Autodesk Inventor part; units mm, degrees
ref_plane "YZ Plane" through (0, 0, 0) normal (1, 0, 0) x (0, 1, 0)
ref_plane "XZ Plane" through (0, 0, 0) normal (0, 1, 0) x (-1, 0, 0)
ref_plane "XY Plane" through (0, 0, 0) normal (0, 0, 1) x (1, 0, 0)
ref_plane "Work Plane6" through (39.7008, -57.1298, -11.5364) normal (0, 0, 1) x (1, 0, 0)
sketch "Sketch1" plane through (39.7008, -57.1298, -11.5364) normal (0, 0, 1) x (1, 0, 0)
  line L0 (-30.146, 63.9369) -> (29.7552, 63.9369)
  line L1 (29.7552, 63.9369) -> (29.7552, 15.006)
  line L2 (29.7552, 15.006) -> (-30.146, 15.006)
  line L3 (-30.146, 15.006) -> (-30.146, 63.9369)
  point P0 (-39.7008, 57.1298)
extrude "Extrusion1" add sketch "Sketch1" against normal blind 3.81
ref_plane "Work Plane5" through (9.5547, -42.1238, -11.5364) normal (0, -1, 0) x (1, 0, 0)
sketch "Sketch4" plane through (9.5547, -42.1238, -11.5364) normal (0, -1, 0) x (1, 0, 0)
  line L0 (59.9013, -3.81) -> (0, -3.81)
  line L1 (51.9539, -3.81) -> (48.6512, -3.81)
  line L2 (48.6512, -3.81) -> (48.6512, -2.9224)
  line L3 (48.6512, -2.9224) -> (51.9539, -2.9224)
  line L4 (51.9539, -2.9224) -> (51.9539, -3.81)
  line L5 (14.0976, -3.7678) -> (10.0617, -3.7678)
  line L6 (10.0617, -3.7678) -> (10.0617, -2.9224)
  line L7 (10.0617, -2.9224) -> (14.0976, -2.9224)
  line L8 (14.0976, -2.9224) -> (14.0976, -3.7678)
  point P0 (-9.5547, 11.5364)
  point P1 (48.6512, -3.81)
extrude "Extrusion2" add sketch "Sketch4" along normal blind 2.54
sketch "Sketch5" plane through (39.7008, -57.1298, -11.5364) normal (0, 0, 1) x (1, 0, 0)
  line L0 (-17.172, 70.4399) -> (-9.7142, 70.4399)
  line L1 (-9.7142, 70.4399) -> (-9.7142, 57.1298)
  line L2 (-9.7142, 57.1298) -> (-17.172, 57.1298)
  line L3 (-17.172, 57.1298) -> (-17.172, 70.4399)
  point P0 (-39.7008, 57.1298)
extrude "Extrusion3" add sketch "Sketch5" along normal blind 2.54
sketch "Sketch6" plane through (39.7008, -57.1298, -8.9964) normal (0, 0, 1) x (1, 0, 0)
  point P0 (-39.7008, 57.1298)
  point P1 (-13.4232, 67.2539)
hole "Hole1" at (26.2775, 10.1241, -8.9964) direction (0, 0, -1) diameter 2.286 end through all
properties part number "batteryFlap"
Read the model definition and answer for the solid it produces. Units are mm, in the model's axes. A direction names the side the tool comes from. Round coordinates to 2 decimals unless told otherwise and drop trailing zeros. Loops run counter-clockwise (first coordinate to the right, second up) from the corner with the lowest first, then second, coordinate; pieces in that order, holes last.
Q1. Which of the six approach directions +Z, -Z, +X, -X, +Y, -Y give full straight-line access (tool end or side, diameter ignored) to faces 1 (the face through (22.529, 7, -10)), 2 (the face through (22, -43, -14.459)), 3 (the face through (25, 9, -11.536)), 4 (the face through (29.987, 7, -10))?
Q2. Each of these flat-tipped pins is pushed along its axis until it touches: pin 1 (2 mm diameter, centred on x = 60.5, y = -44, fed in from +Z); pin 2 (0.9 mm diameter, centred on y = -44, z = -15, fed in from -X); pin 3 (1.5 mm diameter, centred on x = 30.5, z = -12, fed in from -Y); pin 4 (5 mm diameter, centred on x = 49, y = 7, fed in from -Z). Where does it stop, or does it pass through?
Q3. Section A-A on y = 1 is taken. Write down the section's boundary in (x, z).
Q4. Section B-B on z = -10.25 is taken. Write down the section's boundary in (x, y), and give its area (3 significant figures).
Q5. Determine the mould class of faces 5 (the face through (40, -42.124, -13)), 6 (the face through (25.144, 10.273, -10.284)), 7 (the face through (39, -17, -11.536)), 8 (the face through (9.555, -18, -13)) for opening direction X: released by +X, released by -X, zero draft, split by the parting line, or undercut.
Q6. Section C-C on x = 15.5 is taken. Write down the section's boundary in (y, z), and give its area (3 significant figures).
Q7. Consider probe 1 along Y at (x, z) = (61.5, -14); probe 2 along Z at (x, y) = (44, -14.5); probe 3 along Y at (x, z) = (24, -10.25). Determine where each line is inside the solid, lowest interval first.
Output:
1. face 1: +Z, -X, +Y, -Y
1. face 2: +Z, +X, -X, -Y
1. face 3: -Z, +X, -X, +Y
1. face 4: +Z, +X, +Y, -Y
2. pin 1: stops at z = -14.46
2. pin 2: stops at x = 19.62
2. pin 3: stops at y = -42.12
2. pin 4: stops at z = -15.35
3. outline: (9.55, -15.35) - (69.46, -15.35) - (69.46, -11.54) - (29.99, -11.54) - (29.99, -9) - (22.53, -9) - (22.53, -11.54) - (9.55, -11.54) - close
4. outline: (22.53, 0) - (29.99, 0) - (29.99, 13.31) - (22.53, 13.31) - close; hole circle Ø2.29 at (26.28, 10.12)
4. area: 95.2 mm2
5. face 5: undercut
5. face 6: undercut
5. face 7: zero draft
5. face 8: released by -X
6. outline: (-42.12, -15.35) - (6.81, -15.35) - (6.81, -11.54) - (-42.12, -11.54) - close
6. area: 186 mm2
7. probe 1: y = -42.12 to 6.81
7. probe 2: z = -15.35 to -11.54
7. probe 3: y = 0 to 13.31
